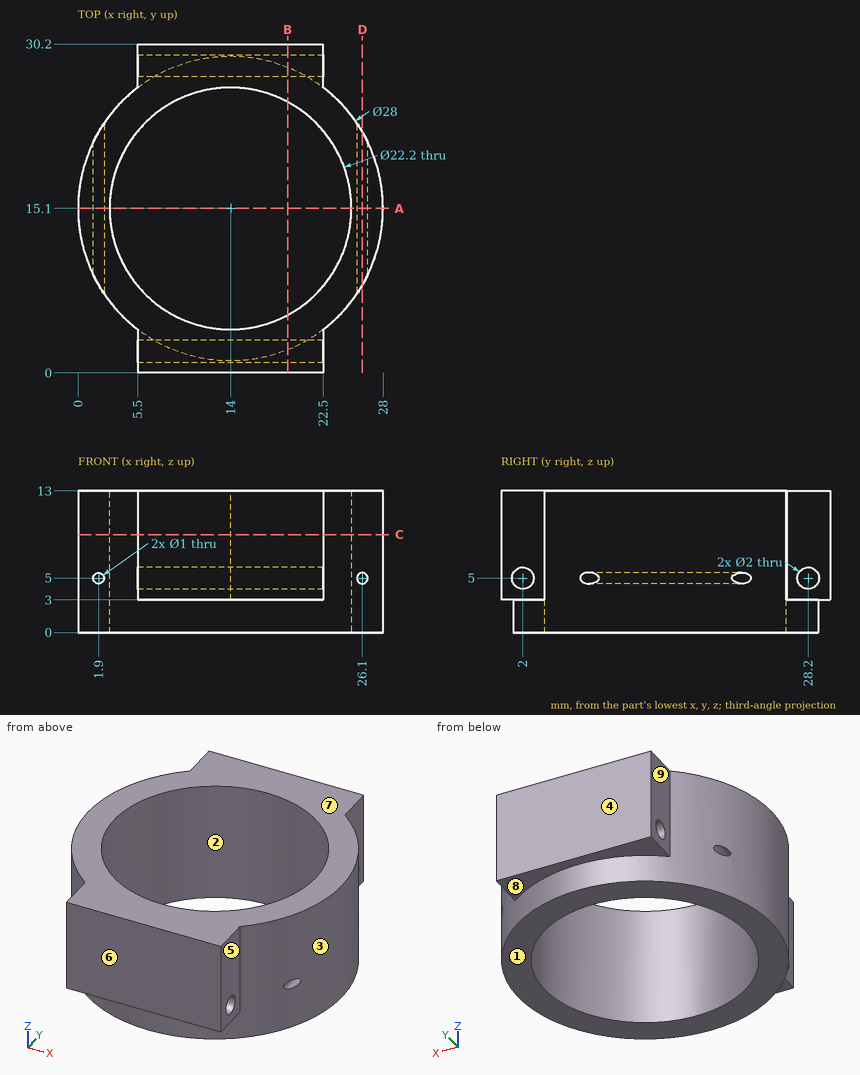
The drawing under review shows one solid part. Ordinate dimensions are in mm from its lowest x, y, z. A direction names the side the tool comes from. Coordinates: 2 decimals unless noted, no trailing zeros. Loops run counter-clockwise (first coordinate to the right, second up) from the corner with the lowest first, then second, coordinate; pieces in that order, holes last.
Item 1: Add section B-B (x = 19.25). Write out the cut boundary in (y, z).
Completed:
outline: (0, 3) - (2.12, 3) - (2.12, 0) - (5.32, 0) - (5.32, 13) - (0, 13) - close; (24.88, 0) - (28.08, 0) - (28.08, 3) - (30.2, 3) - (30.2, 13) - (24.88, 13) - close; hole circle Ø2 at (2, 5); hole circle Ø2 at (28.2, 5)
Item 2: For the marked faces 5, 6, 7, 8 and 9, list the 3-axis set-ups (+Z, -Z, +X, -X, +Y, -Y) from which the entire face can be reached by the end or side of a thin tool; tool diameter is ignored.
Completed:
face 5: +Z, -Z, +X, -Y
face 6: +Z, -Z, +X, -X, -Y
face 7: +Z, +X, -X, +Y, -Y
face 8: -Z, +Y
face 9: +Z, -Z, -X, +Y
Item 3: Add section C-C (z = 9). Write out the cut boundary in (x, y).
Completed:
outline: (5.5, 0) - (22.5, 0) - (22.5, 3.98) arc R14 ccw to (22.5, 26.22) - (22.5, 30.2) - (5.5, 30.2) - (5.5, 26.22) arc R14 ccw to (5.5, 3.98) - close; hole circle Ø22.2 at (14, 15.1)
Item 4: Draft analysis for pull direction Y (two halves, no side actions). For the marked faces 1, 2, 3 and 4, state which applies: pulls with the +Y half, pulls with the -Y half, needs draft (parallel to the pull), parting line crosses it, or undercut.
Completed:
face 1: needs draft
face 2: undercut
face 3: parting line crosses it
face 4: pulls with the +Y half
Item 5: Add section A-A (y = 15.1). Write out the cut boundary in (x, z), and give its area (3 significant figures).
Completed:
outline: (0, 0) - (2.9, 0) - (2.9, 13) - (0, 13) - close; (25.1, 0) - (28, 0) - (28, 13) - (25.1, 13) - close; hole circle Ø1 at (1.9, 5); hole circle Ø1 at (26.1, 5)
area: 73.8 mm2
Item 6: Wall thickness on L1, parallel to Z at x = 13, y = 2; L2, parallel to Y at x = 7.25, z = 4.75; L3, parallel to Z at x = 26.1, y = 15: over which ranges is each line inside the solid? List them lowest first.
Completed:
L1: z = 0 to 4, 6 to 13
L2: y = 0 to 1.03, 2.97 to 6.29, 23.91 to 27.23, 29.17 to 30.2
L3: z = 0 to 4.5, 5.5 to 13
Item 7: Clearance check with flat-ended pins moving along their axes: pin 1 (3 mm diameter, centred on y = 18.5, z = 2.5, fed in from +X); pin 2 (2 mm diameter, centred on y = 28, z = 9.5, fed in from -X); pin 3 (3 mm diameter, centred on y = 29, z = 6.5, fed in from +X); pin 4 (1.2 mm diameter, centred on y = 28.2, z = 5, fed in from +X). State where each tip first meets the part, or that it passes through.
Completed:
pin 1: stops at x = 27.87
pin 2: stops at x = 5.5
pin 3: stops at x = 22.5
pin 4: passes through
Item 8: Add section D-D (x = 26.1). Write out the cut boundary in (y, z), and give its area (3 significant figures).
Completed:
outline: (8.06, 0) - (22.14, 0) - (22.14, 4.5) - (8.06, 4.5) - close; (8.06, 5.5) - (22.14, 5.5) - (22.14, 13) - (8.06, 13) - close
area: 169 mm2
